Work out the finished part from the listing and answer in its coordinate system (mm). Face numbers are marked on the shaded views. A direction names the side the tool comes from. Give positions to 0.01 mm unless a question says otherwise; leave off trailing zeros. Order: outer loops, then holes, each group sorted by start corner. A loop starts at its lowest first (then second) coordinate and runs counter-clockwise, first axis right, second up. Notation, with made-up numbers: (0, 86) - (14, 86) arc R10 ccw to (14, 97) - close; hole circle Ø4 at (-29, 50). An arc over 180 degrees is marked (long way). Put each result on its own line as item: value.
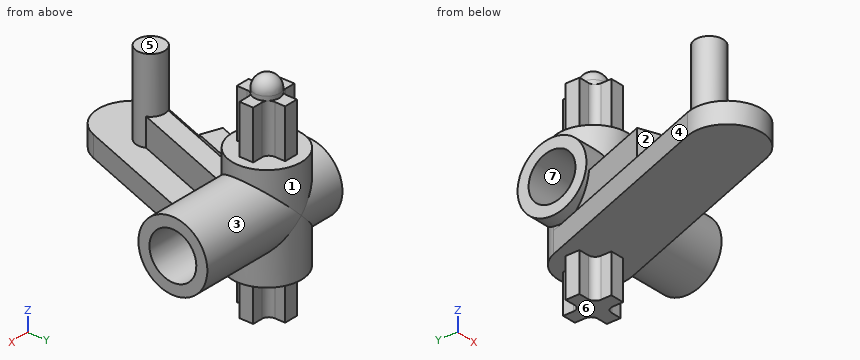
```python
from build123d import *

# Parameters (mm, degrees)
ESTRUSIONE_ESTRUSIONE1_DEPTH  = 1.5
SCHIZZO2_R                    = 2.5
ESTRUSIONE_ESTRUSIONE2_DEPTH  = 7.5
SCHIZZO3_R                    = 1
ESTRUSIONE_ESTRUSIONE3_DEPTH  = 6
SCHIZZO4_R                    = 2.5
ESTRUSIONE_ESTRUSIONE8_DEPTH  = 8
ESTRUSIONE_ESTRUSIONE16_START = -3.5
SCHIZZO5_R                    = 2.5
ESTRUSIONE_ESTRUSIONE16_DEPTH = 3.5
SCHIZZO7_W                    = 1
SCHIZZO7_H                    = 3.5
SCHIZZO7_W_2                  = 3.5
SCHIZZO7_H_2                  = 1
ESTRUSIONE_SOTTILE1_DEPTH     = 3.5
RACCORDO1_R                   = 0.5
RACCORDO1_OF_SPECCHIA6_R      = 0.5
SCHIZZO10_R                   = 0.914213562
ESTRUSIONE_ESTRUSIONE17_DEPTH = 0.3
ESTRUSIONE_ESTRUSIONE18_DEPTH = 2.2
ESTRUSIONE_ESTRUSIONE19_DEPTH = 2
FORO_PER_VITE_M3_1_D          = 3.4


with BuildPart() as part:
    # Schizzo1 → Estrusione-Estrusione1 (new body)
    with BuildSketch(Plane.XY):
        with BuildLine():
            Line((2.349231552, -0.855050358), (-2.781070598, -14.95043967))
            ThreePointArc((-2.781070598, -14.95043967), (-5.985352508, -16.444620864), (-7.479533702, -13.240338953))
            Line((-7.479533702, -13.240338953), (-2.349231552, 0.855050358))
            ThreePointArc((-2.349231552, 0.855050358), (0.855050358, 2.349231552), (2.349231552, -0.855050358))
        make_face()
    extrude(amount=ESTRUSIONE_ESTRUSIONE1_DEPTH)

    # Schizzo2 → Estrusione-Estrusione2 (add)
    with BuildSketch(Plane.XY):
        with Locations(Location((0, 0, 0), (0, 0, 160))):
            Circle(SCHIZZO2_R)
    extrude(amount=ESTRUSIONE_ESTRUSIONE2_DEPTH)

    # Schizzo3 → Estrusione-Estrusione3 (add)
    with BuildSketch(Plane.XY.offset(1.5)):
        with Locations((-4.446261863, -12.21600407)):
            Circle(SCHIZZO3_R)
    extrude(amount=ESTRUSIONE_ESTRUSIONE3_DEPTH)

    # Schizzo4 → Estrusione-Estrusione8 (add)
    with BuildSketch(Plane(origin=(0, 0, 0), x_dir=(0, 0, -1), z_dir=(1, 0, 0))):
        with Locations(Location((-4.1, 0, 0), (0, 0, 270))):
            Circle(SCHIZZO4_R)
    extrude(amount=ESTRUSIONE_ESTRUSIONE8_DEPTH)

    # Schizzo5 → Estrusione-Estrusione16 (add)
    with BuildSketch(Plane(origin=(0, 0, 0), x_dir=(0, 0, -1), z_dir=(1, 0, 0)).offset(ESTRUSIONE_ESTRUSIONE16_START)):
        with Locations(Location((-4.1, 0, 0), (0, 0, 270))):
            Circle(SCHIZZO5_R)
    extrude(amount=ESTRUSIONE_ESTRUSIONE16_DEPTH)

    # Schizzo7 → Estrusione-Sottile1 (add)
    with BuildSketch(Plane.XY.offset(7.5)):
        Rectangle(SCHIZZO7_W, SCHIZZO7_H)
        Rectangle(SCHIZZO7_W_2, SCHIZZO7_H_2)
    estrusione_sottile1 = extrude(amount=ESTRUSIONE_SOTTILE1_DEPTH)

    # Raccordo1
    raccordo1_edges = [part.edges().sort_by_distance(p)[0] for p in [
        (-0.5, 0.5, 9.25),
        (0.5, -0.5, 9.25),
        (-0.5, -0.5, 9.25),
        (0.5, 0.5, 9.25),
    ]]
    fillet(raccordo1_edges, radius=RACCORDO1_R)

    # Specchia6: Estrusione-Sottile1 across plane
    add(estrusione_sottile1.mirror(Plane.XY.offset(4.1)))

    # Raccordo1 of Specchia6
    raccordo1_of_specchia6_edges = [part.edges().sort_by_distance(p)[0] for p in [
        (-0.5, 0.5, -1.05),
        (0.5, -0.5, -1.05),
        (-0.5, -0.5, -1.05),
        (0.5, 0.5, -1.05),
    ]]
    fillet(raccordo1_of_specchia6_edges, radius=RACCORDO1_OF_SPECCHIA6_R)

    # Schizzo10 → Estrusione-Estrusione17 (add)
    with BuildSketch(Plane.XY.offset(11)):
        with Locations(Location((0, 0, 0), (0, 0, 135))):
            Circle(SCHIZZO10_R)
    extrude(amount=ESTRUSIONE_ESTRUSIONE17_DEPTH)

    # Schizzo11 → Rivoluzione2 (revolve)
    with BuildSketch(Plane.XY.offset(11.3)):
        with BuildLine():
            Line((-0.914213562, 0), (0.914213562, 0))
            ThreePointArc((0.914213562, 0), (0, 0.914213562), (-0.914213562, 0))
        make_face()
    revolve(axis=Axis((-0.914213562, 0, 11.3), (1, 0, 0)))

    # Schizzo12 → Estrusione-Estrusione18 (add)
    with BuildSketch(Plane.XY.offset(1.5)):
        Polygon((-5.077352246, -7.517540966), (-2.341191099, 0), (-0.931652168, -0.513030215), (-3.667813315, -8.030571181), align=None)
    extrude(amount=ESTRUSIONE_ESTRUSIONE18_DEPTH)

    # Schizzo13 → Estrusione-Estrusione19 (add)
    with BuildSketch(Plane.XY.offset(1.5)):
        Polygon((-3.788477029, -12.455418171), (0.744924441, 0), (-0.744924441, 0), (-5.104046698, -11.97658997), align=None)
    extrude(amount=ESTRUSIONE_ESTRUSIONE19_DEPTH)

    # Foro per Vite M3-1 (through all)
    with Locations(Plane(origin=(-3.5, 0, 4.1), x_dir=(0, 0, -1), z_dir=(-1, 0, 0))):
        with Locations((0, 0)):
            Hole(FORO_PER_VITE_M3_1_D / 2)


solid = part.part
```
(1) A tool of negligible diameter and unlimited length cuts with its end or side. For the marked faces 1, 2 and 3, from which of +Z, -Z, +X, -X, +Y, -Y can it reach the whole face along a straight path? Write none if from no direction.
Geometry check:
face 1: +Z
face 2: +Z, -X
face 3: +X
(2) Section B-B, the plane z = 9.5 is taken. Write down the section's boundary in (x, y), then the cut area to 3 significant figures.
Geometry check:
outline: (-1.75, -0.5) - (-1, -0.5) arc R0.5 cw to (-0.5, -1) - (-0.5, -1.75) - (0.5, -1.75) - (0.5, -1) arc R0.5 cw to (1, -0.5) - (1.75, -0.5) - (1.75, 0.5) - (1, 0.5) arc R0.5 cw to (0.5, 1) - (0.5, 1.75) - (-0.5, 1.75) - (-0.5, 1) arc R0.5 cw to (-1, 0.5) - (-1.75, 0.5) - close
area: 6.21 mm²
(3) Determine the mould class of the marked faces 4, 5, 6 and 7 for opening direction Z: pulls with the +Z half, pulls with the -Z half, needs draft (parallel to the pull), parting line crosses it, or undercut.
Geometry check:
face 4: needs draft
face 5: pulls with the +Z half
face 6: pulls with the -Z half
face 7: undercut
(4) Straight lines are drawn through the part: line 1 (X direction, y = 0, z = -1.5); line 2 (X direction, y = -12, z = 5); line 3 (Y direction, x = -0.75, z = 9.5). For each, find the intervals that lie inside material, in ascending order.
Geometry check:
line 1: x = -1.75 to 1.75
line 2: x = -5.42 to -3.47
line 3: y = -0.57 to 0.57
(5) Given pin 1 (0.8 mm diameter, centred on y = 1.5, z = 9.5, fed in from +X); pin 2 (0.5 mm diameter, centred on y = 0, z = 10, fed in from +X); pin 3 (1.2 mm diameter, centred on x = 0.5, y = 1.5, fed in from +Z); pin 4 (2 mm diameter, centred on y = 0, z = 4.1, fed in from -X), each flat-ended and moving along its own axis, determine where each tip first touches the part or whether it passes through.
Geometry check:
pin 1: stops at x = 0.5
pin 2: stops at x = 1.75
pin 3: stops at z = 11
pin 4: passes through
(6) Section D-D, the plane y = -6 is taken. Write down the section's boundary in (x, z), then the cut area to 3 significant figures.
Geometry check:
outline: (-4.84, 0) - (0.48, 0) - (0.48, 1.5) - (-1.44, 1.5) - (-1.44, 3.5) - (-2.93, 3.5) - (-2.93, 3.7) - (-4.53, 3.7) - (-4.53, 1.5) - (-4.84, 1.5) - close
area: 14.5 mm²
(7) Section C-C, the plane x = 5.25 is taken. Write down the section's boundary in (y, z), then the cut area to 3 significant figures.
Geometry check:
outline: circle Ø5 at (0, 4.1); hole circle Ø3.4 at (0, 4.1)
area: 10.6 mm²
